```python
from build123d import *

# Parameters (mm, degrees)
SKETCH1_W         = 30.9626
SKETCH1_H         = 17.0688
EXTRUDE1_DEPTH    = 41.6814
SKETCH3_OUTSIDE_W = 43.895
SKETCH3_OUTSIDE_H = 30.001
EXTRUDE2_DEPTH    = 42.6814
SKETCH4_W         = 6.35
SKETCH4_H         = 17.0688
EXTRUDE3_DEPTH    = 6.35
SKETCH5_W         = 6.35
SKETCH5_H         = 7.239
EXTRUDE4_DEPTH    = 1.5748
SKETCH6_W         = 28.9814
SKETCH6_H         = 15.494
EXTRUDE5_DEPTH    = 1.5748
SKETCH7_W         = 1.6002
SKETCH7_H         = 1.5748
SKETCH7_W_2       = 1.5748
EXTRUDE6_DEPTH    = 10.3124
FILLET1_R         = 1.5875
FILLET2_R         = 0.254
SKETCH8_R         = 4.0005
SKETCH8_R_2       = 1.1938
EXTRUDE7_DEPTH    = 1.5748
SKETCH9_R         = 1.5875
EXTRUDE9_DEPTH    = 31.9626
FILLET3_R         = 2.54


with BuildPart() as part:
    # Sketch1 → Extrude1 (new body)
    with BuildSketch(Plane(origin=(0, 0, 0), x_dir=(0, 0, -1), z_dir=(1, 0, 0))):
        with Locations((15.4813, 8.5344)):
            Rectangle(SKETCH1_W, SKETCH1_H)
    extrude(amount=EXTRUDE1_DEPTH)

    # Sketch3 outside → Extrude2 (cut, through all)
    with BuildSketch(Plane(origin=(41.6814, 0, 0), x_dir=(0, 0, -1), z_dir=(1, 0, 0))):
        with Locations((15.4815, 8.5345)):
            Rectangle(SKETCH3_OUTSIDE_W, SKETCH3_OUTSIDE_H)
        Polygon((0, 17.0688), (0, 0), (30.9626, 0), (30.9626, 1.5748), (23.7236, 1.5748), (23.7236, 17.0688), (22.1488, 17.0688), (22.1488, 1.5748), (1.5748, 1.5748), (1.5748, 17.0688), align=None, mode=Mode.SUBTRACT)
    extrude(amount=-EXTRUDE2_DEPTH, mode=Mode.SUBTRACT)

    # Sketch4 → Extrude3 (cut)
    with BuildSketch(Plane.XY):
        with Locations((3.175, 8.5344)):
            Rectangle(SKETCH4_W, SKETCH4_H)
        with Locations((38.5064, 8.5344)):
            Rectangle(SKETCH4_W, SKETCH4_H)
    extrude(amount=-EXTRUDE3_DEPTH, mode=Mode.SUBTRACT)

    # Sketch5 → Extrude4 (cut)
    with BuildSketch(Plane(origin=(0, 1.5748, 0), x_dir=(1, 0, 0), z_dir=(0, 1, 0))):
        with Locations((3.175, 27.3431)):
            Rectangle(SKETCH5_W, SKETCH5_H)
        with Locations((38.5064, 27.3431)):
            Rectangle(SKETCH5_W, SKETCH5_H)
    extrude(amount=-EXTRUDE4_DEPTH, mode=Mode.SUBTRACT)

    # Sketch6 → Extrude5 (cut)
    with BuildSketch(Plane(origin=(0, 0, -23.7236), x_dir=(-1, 0, 0), z_dir=(0, 0, -1))):
        with Locations((-20.8407, 9.3218)):
            Rectangle(SKETCH6_W, SKETCH6_H)
    extrude(amount=-EXTRUDE5_DEPTH, mode=Mode.SUBTRACT)

    # Sketch7 → Extrude6 (cut)
    with BuildSketch(Plane(origin=(0, 0, -30.9626), x_dir=(-1, 0, 0), z_dir=(0, 0, -1))):
        with Locations((-34.5313, 0.7874)):
            Rectangle(SKETCH7_W, SKETCH7_H)
        with Locations((-7.1374, 0.7874)):
            Rectangle(SKETCH7_W_2, SKETCH7_H)
    extrude(amount=-EXTRUDE6_DEPTH, mode=Mode.SUBTRACT)

    # Fillet1
    fillet1_edges = [part.edges().sort_by_distance(p)[0] for p in [
        (3.175, 0, -23.7236),
        (38.5064, 0, -23.7236),
        (20.8407, 0, 0),
    ]]
    fillet(fillet1_edges, radius=FILLET1_R)

    # Fillet2
    fillet2_edges = [part.edges().sort_by_distance(p)[0] for p in [
        (38.5064, 1.5748, -22.1488),
        (3.175, 1.5748, -22.1488),
        (20.8407, 1.5748, -1.5748),
    ]]
    fillet(fillet2_edges, radius=FILLET2_R)

    # Sketch8 → Extrude7 (cut)
    with BuildSketch(Plane(origin=(0, 1.5748, 0), x_dir=(1, 0, 0), z_dir=(0, 1, 0))):
        with Locations(Location((12.4968, 18.669, 0), (0, 0, 270))):  # turned: the seam where the file's is
            Circle(SKETCH8_R)
        with Locations(Location((18.7452, 18.669, 0), (0, 0, 270))):  # turned: the seam where the file's is
            Circle(SKETCH8_R_2)
        with Locations(Location((6.2484, 18.669, 0), (0, 0, 270))):  # turned: the seam where the file's is
            Circle(SKETCH8_R_2)
        with Locations(Location((22.9108, 18.669, 0), (0, 0, 270))):  # turned: the seam where the file's is
            Circle(SKETCH8_R_2)
        with Locations(Location((29.1592, 18.669, 0), (0, 0, 270))):  # turned: the seam where the file's is
            Circle(SKETCH8_R)
        with Locations(Location((35.4076, 18.669, 0), (0, 0, 270))):  # turned: the seam where the file's is
            Circle(SKETCH8_R_2)
        with BuildLine():
            Line((13.6906, 27.0002), (13.6906, 24.9174))
            ThreePointArc((13.6906, 24.9174), (12.4968, 23.7236), (11.303, 24.9174))
            Line((11.303, 24.9174), (11.303, 27.0002))
            ThreePointArc((11.303, 27.0002), (12.4968, 28.194), (13.6906, 27.0002))
        make_face()
        with BuildLine():
            Line((13.6906, 12.3952), (13.6906, 10.3124))
            ThreePointArc((13.6906, 10.3124), (12.4968, 9.1186), (11.303, 10.3124))
            Line((11.303, 10.3124), (11.303, 12.3952))
            ThreePointArc((11.303, 12.3952), (12.4968, 13.589), (13.6906, 12.3952))
        make_face()
        with BuildLine():
            Line((27.9654, 12.3952), (27.9654, 10.3124))
            ThreePointArc((27.9654, 10.3124), (29.1592, 9.1186), (30.353, 10.3124))
            Line((30.353, 10.3124), (30.353, 12.3952))
            ThreePointArc((30.353, 12.3952), (29.1592, 13.589), (27.9654, 12.3952))
        make_face()
        with BuildLine():
            Line((27.9654, 27.0002), (27.9654, 24.9174))
            ThreePointArc((27.9654, 24.9174), (29.1592, 23.7236), (30.353, 24.9174))
            Line((30.353, 24.9174), (30.353, 27.0002))
            ThreePointArc((30.353, 27.0002), (29.1592, 28.194), (27.9654, 27.0002))
        make_face()
    extrude(amount=-EXTRUDE7_DEPTH, mode=Mode.SUBTRACT)

    # Sketch9 → Extrude9 (cut, through all)
    with BuildSketch(Plane.XY):
        with Locations(Location((2.7686, 10.3124, 0), (0, 0, 270))):  # turned: the seam where the file's is
            Circle(SKETCH9_R)
        with Locations((12.7, 10.3124)):
            Circle(SKETCH9_R)
        with Locations((28.9814, 10.3124)):
            Circle(SKETCH9_R)
        with Locations(Location((38.8874, 10.3124, 0), (0, 0, 270))):  # turned: the seam where the file's is
            Circle(SKETCH9_R)
    extrude(amount=-EXTRUDE9_DEPTH, mode=Mode.SUBTRACT)

    # Fillet3
    fillet3_edges = [part.edges().sort_by_distance(p)[0] for p in [
        (6.35, 17.0688, -22.9362),
        (35.3314, 17.0688, -22.9362),
        (0, 17.0688, -22.9362),
        (33.7312, 0.7874, -30.9626),
        (7.9248, 0.7874, -30.9626),
        (41.6814, 17.0688, -22.9362),
        (0, 0.7874, -6.35),
        (6.35, 17.0688, -0.7874),
        (35.3314, 17.0688, -0.7874),
        (41.6814, 0.7874, -6.35),
    ]]
    fillet(fillet3_edges, radius=FILLET3_R)


solid = part.part
```
The model under review builds one solid part; all positions refer to its coordinate system, in mm. A direction names the side the tool comes from. Round coordinates to 2 decimals unless told otherwise and drop trailing zeros. Loops run counter-clockwise (first coordinate to the right, second up) from the corner with the lowest first, then second, coordinate; pieces in that order, holes last.
1) The part is to be moulded in two halves that separate along X. For faces 1 (the face through (15.87, 0.8, -16.52)), 2 (the face through (6.35, 6, -1)), 3 (the face through (5, 10, -22.149)), say which applies: pulls with the +X half, pulls with the -X half, needs draft (parallel to the pull), parting line crosses it, or undercut.
Values follow:
face 1: undercut
face 2: pulls with the -X half
face 3: needs draft
2) Tool access review of faces 4 (the face through (4, 1, -6.35)), 5 (the face through (37, 10, -22.149)), 6 (the face through (29.13, 0.8, -9.12)), 7 (the face through (35, 1, -20.65)), 8 (the face through (21, 9, -1.575)): name each direction out of +Z, -Z, +X, -X, +Y, -Y from which nothing blocks a thin tool from reaching the whole face with its end or side.
Values follow:
face 4: +Z, -X, +Y, -Y
face 5: +Z, +X, -X, +Y
face 6: +Y, -Y
face 7: -Z, +Y, -Y
face 8: -Z, +X, -X, +Y
3) Consider section C-C on y = 11. State the section outline as (x, z) points, then the cut area to 3 significant figures.
Values follow:
outline: (0, -23.72) - (1.34, -23.72) - (1.34, -22.15) - (0, -22.15) - close; (4.2, -23.72) - (6.35, -23.72) - (6.35, -22.15) - (4.2, -22.15) - close; (6.35, -1.57) - (11.27, -1.57) - (11.27, 0) - (6.35, 0) - close; (14.13, -1.57) - (27.55, -1.57) - (27.55, 0) - (14.13, 0) - close; (30.41, -1.57) - (35.33, -1.57) - (35.33, 0) - (30.41, 0) - close; (35.33, -23.72) - (37.46, -23.72) - (37.46, -22.15) - (35.33, -22.15) - close; (40.32, -23.72) - (41.68, -23.72) - (41.68, -22.15) - (40.32, -22.15) - close
area: 47.6 mm2
4) Clearance check with flat-ended pins moving along their axes: P1, Ø4, axis at x = 28.98, y = 10.31, coming from the -Z side; P2, Ø1.7, axis at y = 1, z = -26, coming from the +X side; P3, Ø1, axis at x = 17, z = -11, coming from the +Y side; P4, Ø2, axis at x = 18.75, z = -18.67, coming from the -Y side. State where each tip first meets the part, or that it passes through.
Values follow:
P1: stops at z = -1.57
P2: stops at x = 33.73
P3: stops at y = 1.57
P4: passes through
5) Consider section D-D on z = -3.5. State the section outline as (x, y) points.
Values follow:
outline: (6.35, 0) - (35.33, 0) - (35.33, 1.57) - (6.35, 1.57) - close
6) Consider section A-A on y = 5. State the section outline as (x, z) points.
Values follow:
outline: (0, -23.72) - (6.35, -23.72) - (6.35, -22.15) - (0, -22.15) - close; (6.35, -1.57) - (35.33, -1.57) - (35.33, 0) - (6.35, 0) - close; (35.33, -23.72) - (41.68, -23.72) - (41.68, -22.15) - (35.33, -22.15) - close
7) Consider section B-B on z = -11.5. State the section outline as (x, y) points, then the cut area to 3 significant figures.
Values follow:
outline: (0, 0) - (11.3, 0) - (11.3, 1.57) - (0, 1.57) - close; (13.69, 0) - (27.97, 0) - (27.97, 1.57) - (13.69, 1.57) - close; (30.35, 0) - (41.68, 0) - (41.68, 1.57) - (30.35, 1.57) - close
area: 58.1 mm2
8) Wall thickness on line 1 along X through (y, z) = (1.25, -12); line 2 along X through (y, z) = (1, -25.5); line 3 along Z through (x, y) = (31, 7): over which ranges is each line inside the solid? List them lowest first.
Values follow:
line 1: x = 0 to 11.3, 13.69 to 27.97, 30.35 to 41.68
line 2: x = 7.92 to 11.3, 13.69 to 27.97, 30.35 to 33.73
line 3: z = -1.57 to 0
